Geometry: final body of the model. Coordinates: model frame, mm. A direction names the side the tool comes from. Round coordinates to 2 decimals unless told otherwise and drop trailing zeros. Write each loop counter-clockwise with the first axis right and the second up, starting at its lowest first coordinate (ties: lowest second). Pieces come first, ordered by that corner, then holes. Notation, with made-up numbers: M 66,-25 L 117,-25 A36 cw 117,13 Z; hole C 36.5,14.25 d8. An arc over 180 degrees is marked long. Use one line per item in the form item = value. Start each with the question number.
Item 1: Section query B-B (y = 106). Return loops of the section in (x, z), and give its area (3 significant figures).
Item 2: Pin query (flat end, axial travel): pin 1 Ø2 at (y, z) = (105, 180.5) entering from +X; pin 2 Ø8 at (x, y) = (36.5, 100.5) entering from -Z; pin 3 Ø6.5 at (y, z) = (127.5, 197) entering from +X. Return the tip coordinate at first contact, or that it passes through.
Item 3: Reachability of faces 1 (the cylindrical face through (30.279, 128.958, 210.686)), 2 (the flat face through (30.2, 111.2, 198.7)), 3 (the flat face through (43, 129, 201)) from +Z, -Z, +X, -X, +Y, -Y: full face, straight path, thin tool, end or side. Return the list, or none.
Item 4: Section query A-A (z = 209). Return loops of the section in (x, y).
Item 5: Ray query, probe 1 along X at (y, z) = (128, 199); probe 2 along X at (y, z) = (130, 209); probe 3 along Z at (x, y) = (49.5, 100). Return the intervals inside material, ascending.
Item 6: Pull-direction query (Z, two-part tool) for faces 4 (the flat face through (28, 129, 204)), 5 (the flat face through (51.305, 114.252, 177.378)), 6 (the cylindrical face through (31.054, 123.651, 197.748)); classes: pulls with the +Z half, pulls with the -Z half, needs draft (parallel to the pull), parting line crosses it, or undercut.
Item 7: Section query D-D (x = 40). State how many separate pieces and enclosed holes the cut face has, and give its area (3 significant figures).
Item 8: Section query C-C (y = 127). Return loops of the section in (x, z).
from build123d import *

# Parameters (mm, degrees)
PAD040_DEPTH    = 6
PAD041_DEPTH    = 30
SKETCH118_R     = 14
POCKET038_DEPTH = 21.001
SKETCH119_R     = 1.7
HOLE023_DEPTH   = 25
SKETCH120_R     = 1.7
HOLE024_DEPTH   = 25


with BuildPart() as part:
    # Sketch116 → Pad040 (new body)
    with BuildSketch(Plane.XZ):
        Polygon((28, 211.5), (43, 211.5), (43, 189.985281), (53.455844, 179.529437), (49.213203, 175.286797), (28, 196.5), align=None)
    extrude(amount=PAD040_DEPTH)

    # Sketch117 (on Face8 of Pad040) → Pad041 (join)
    with BuildSketch(Plane.XZ.offset(6)):
        Polygon((28, 196.5), (49.213203, 175.286797), (53.455844, 179.529437), (32.242641, 200.742641), align=None)
    extrude(amount=PAD041_DEPTH)

    # Sketch118 (on Face10 of Pad041) → Pocket038 (cut, through all)
    with BuildSketch(Plane(origin=(116.492641, 0, 116.492641), x_dir=(-0.707107, 0, 0.707107), z_dir=(0.707107, 0, 0.707107))):
        with Locations((104.206258, 21)):
            Circle(SKETCH118_R)
    extrude(amount=-POCKET038_DEPTH, mode=Mode.SUBTRACT)

    # Sketch119 (on Face10 of Pocket038) → Hole023 (cut)
    with BuildSketch(Plane(origin=(116.492641, 0, 116.492641), x_dir=(-0.707107, 0, 0.707107), z_dir=(0.707107, 0, 0.707107))):
        with Locations((92.3, 33)):
            Circle(SKETCH119_R)
        with Locations((116.3, 33)):
            Circle(SKETCH119_R)
        with Locations((92.3, 9)):
            Circle(SKETCH119_R)
        with Locations((116.3, 9)):
            Circle(SKETCH119_R)
    extrude(amount=-HOLE023_DEPTH, mode=Mode.SUBTRACT)

    # Sketch120 (on Face5 of Hole023) → Hole024 (cut)
    with BuildSketch(Plane.XZ.offset(6)):
        with Locations((30.5, 209)):
            Circle(SKETCH120_R)
        with Locations((40.5, 199)):
            Circle(SKETCH120_R)
    extrude(amount=-HOLE024_DEPTH, mode=Mode.SUBTRACT)


with BuildPart() as part_1:
    # Body017 placement: moved
    add(part.part.moved(Location((0, 132, 0))))


solid = part_1.part
Working result:
q1.outline = M 28,196.5 L 29.32,195.18 L 33.56,199.42 L 32.24,200.74 Z; M 47.81,176.69 L 49.21,175.29 L 53.46,179.53 L 52.05,180.93 Z
q1.area = 23.1 mm²
q2.pin_1 = 53.46
q2.pin_2 = 186.06
q2.pin_3 = 43
q3.face_1 = +Y, -Y
q3.face_2 = +Z, -X, -Y
q3.face_3 = +Z, +X, +Y, -Y
q4.outline = M 28,126 L 28.8,126 L 28.8,132 L 28,132 Z; M 32.2,126 L 43,126 L 43,132 L 32.2,132 Z
q5.probe_1 = 28 to 38.8, 42.2 to 43
q5.probe_2 = 28 to 28.8, 32.2 to 43
q5.probe_3 = 175.57 to 178.09, 181.98 to 183.49
q6.face_4 = needs draft
q6.face_5 = pulls with the -Z half
q6.face_6 = undercut
q7.separate_pieces = 3
q7.enclosed_holes = 0
q7.area = 162 mm²
q8.outline = M 28,196.5 L 49.21,175.29 L 53.46,179.53 L 43,189.99 L 43,211.5 L 28,211.5 Z; hole C 30.5,209 d3.4; hole C 40.5,199 d3.4
